Work out the finished part from the listing and answer in its coordinate system (mm). Face numbers are marked on the shaded views. A direction names the side the tool comes from. Coordinates: 2 decimals unless noted, no trailing zeros. Loops run counter-clockwise (first coordinate to the right, second up) from the corner with the lowest first, then second, coordinate; pieces in that order, holes last. Notation, with made-up numbers: M 61,-3.75 L 86,-3.75 A22 cw 86,9.25 Z; hole C 27,-29.5 d2. An arc over 180 degrees is marked long. Write each question's results on one line, items separated by ' | '.
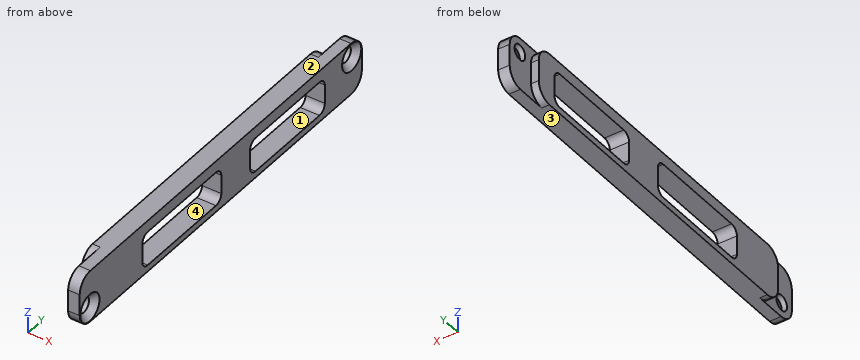
Autodesk Inventor part; units mm, degrees
ref_plane "YZ Plane" through (0, 0, 0) normal (1, 0, 0) x (0, 1, 0)
ref_plane "XZ Plane" through (0, 0, 0) normal (0, 1, 0) x (-1, 0, 0)
ref_plane "XY Plane" through (0, 0, 0) normal (0, 0, 1) x (1, 0, 0)
sketch "Sketch1" plane through (0, 0, 0) normal (1, 0, 0) x (0, 1, 0)
  line L0 (2, 0) -> (50.8, 0)
  line L1 (52.8, -2) -> (52.8, -4.8)
  line L2 (50.8, -6.8) -> (2, -6.8)
  line L3 (0, -4.8) -> (0, -2)
  arc A0 (2, 0) -> (0, -2) centre (2, -2) ccw
  arc A1 (0, -4.8) -> (2, -6.8) centre (2, -4.8) ccw
  arc A2 (50.8, -6.8) -> (52.8, -4.8) centre (50.8, -4.8) ccw
  arc A3 (52.8, -2) -> (50.8, 0) centre (50.8, -2) ccw
  line L4 (26.4, 0) -> (26.4, -6.5481) construction
  line L5 (52.8, -3.4) -> (39.7965, -3.4) construction
  circle A4 centre (1.9, -4.9) radius 1
  circle A5 centre (50.9, -4.9) radius 1 construction
  circle A6 centre (50.9, -1.9) radius 1
  point P0 (0, 0)
  point P1 (52.8, 0)
  point P2 (0, -6.8)
  dimension "d0" = 52.8
  dimension "d1" = 6.8
  dimension "d2" = 2
  dimension "d19" = 2
  dimension "d20" = 0.1
  dimension "d21" = 0.1
extrude "Extrusion1" add sketch "Sketch1" along normal blind 1.5
chamfer "Chamfer1" distance 0.8 angle 45 2 edges at (1.5, 49.9, -1.9) (1.5, 0.9, -4.9)
sketch "Sketch2" plane through (1.5, 0, 0) normal (1, 0, 0) x (0, 0, -1)
  line L0 (0, 50.8) -> (0, 2)
  line L1 (2.5, 45.871) -> (4.9546, 45.871)
  line L2 (5.9546, 44.871) -> (5.9546, 32.8996)
  line L3 (4.9546, 31.8996) -> (2.5, 31.8996)
  line L4 (1.5, 32.8996) -> (1.5, 44.871)
  line L5 (2.5, 26.5) -> (4.9546, 26.5)
  line L6 (5.9546, 25.5) -> (5.9546, 12.7187)
  line L7 (4.9546, 11.7187) -> (2.5, 11.7187)
  line L8 (1.5, 12.7187) -> (1.5, 25.5)
  arc A0 (5.9546, 44.871) -> (4.9546, 45.871) centre (4.9546, 44.871) ccw
  arc A1 (2.5, 45.871) -> (1.5, 44.871) centre (2.5, 44.871) ccw
  arc A2 (1.5, 32.8996) -> (2.5, 31.8996) centre (2.5, 32.8996) ccw
  arc A3 (4.9546, 31.8996) -> (5.9546, 32.8996) centre (4.9546, 32.8996) ccw
  arc A4 (5.9546, 25.5) -> (4.9546, 26.5) centre (4.9546, 25.5) ccw
  arc A5 (4.9546, 11.7187) -> (5.9546, 12.7187) centre (4.9546, 12.7187) ccw
  arc A6 (1.5, 12.7187) -> (2.5, 11.7187) centre (2.5, 12.7187) ccw
  arc A7 (2.5, 26.5) -> (1.5, 25.5) centre (2.5, 25.5) ccw
  point P0 (0, 0)
  dimension "d9" = 1
  dimension "d10" = 1.5
  dimension "d11" = 1.5
extrude "Extrusion2" cut sketch "Sketch2" against normal blind 1.5
sketch "Sketch3" plane through (0, 0, 0) normal (-1, 0, 0) x (0, 0, 1)
  arc A0 (-1.5, 44.871) -> (-2.5, 45.871) centre (-2.5, 44.871) ccw
  line L0 (-1.5, 44.871) -> (-1.5, 32.8996)
  arc A1 (-2.5, 31.8996) -> (-1.5, 32.8996) centre (-2.5, 32.8996) ccw
  line L1 (-2.5, 31.8996) -> (-4.9546, 31.8996)
  arc A2 (-5.9546, 32.8996) -> (-4.9546, 31.8996) centre (-4.9546, 32.8996) ccw
  line L2 (-5.9546, 32.8996) -> (-5.9546, 44.871)
  arc A3 (-4.9546, 45.871) -> (-5.9546, 44.871) centre (-4.9546, 44.871) ccw
  line L3 (-4.9546, 45.871) -> (-2.5, 45.871)
  arc A4 (-4.9546, 26.5) -> (-5.9546, 25.5) centre (-4.9546, 25.5) ccw
  line L4 (-4.9546, 26.5) -> (-2.5, 26.5)
  arc A5 (-1.5, 25.5) -> (-2.5, 26.5) centre (-2.5, 25.5) ccw
  line L5 (-1.5, 25.5) -> (-1.5, 12.7187)
  arc A6 (-2.5, 11.7187) -> (-1.5, 12.7187) centre (-2.5, 12.7187) ccw
  line L6 (-2.5, 11.7187) -> (-4.9546, 11.7187)
  arc A7 (-5.9546, 12.7187) -> (-4.9546, 11.7187) centre (-4.9546, 12.7187) ccw
  line L7 (-5.9546, 12.7187) -> (-5.9546, 25.5)
  line L8 (0, 50.8) -> (0, 2)
  line L9 (-4.8, 52.8) -> (-2, 52.8)
  line L10 (-4.8, 48.8) -> (-2, 48.8)
  line L11 (0, 46.8) -> (0, 6)
  line L12 (-2, 4) -> (-4.8, 4)
  line L13 (-6.8, 6) -> (-6.8, 46.8)
  arc A8 (-4.8, 48.8) -> (-6.8, 46.8) centre (-4.8, 46.8) ccw
  arc A9 (0, 46.8) -> (-2, 48.8) centre (-2, 46.8) ccw
  arc A10 (-2, 4) -> (0, 6) centre (-2, 6) ccw
  arc A11 (-6.8, 6) -> (-4.8, 4) centre (-4.8, 6) ccw
  line L14 (-3.4, 52.8) -> (-3.4, 49.069) construction
  line L15 (-3.4, 48.8) -> (-3.4, 44.871) construction
  line L16 (0, 26.4) -> (-3, 26.4) construction
  line L17 (-6.8, 26.4) -> (-12.1303, 26.4) construction
  point P0 (0, 0)
  point P1 (0, 4)
  point P2 (0, 48.8)
  point P3 (-6.8, 4)
  point P4 (-6.8, 45.8508)
  point P5 (-6.8, 31.9198)
  point P6 (-6.8, 26.4798)
  point P7 (-6.8, 11.7389)
  dimension "d14" = 6.8
  dimension "d15" = 44.8
  dimension "d16" = 2
extrude "Extrusion3" add sketch "Sketch3" along normal blind 1
properties part number "IOModulePlate01"
1) Given pin 1 Ø1.8 at (y, z) = (50, -3.5) entering from -X; pin 2 Ø1.5 at (x, z) = (-0.5, -6) entering from -Y, each flat-ended and moving along its own axis, determine where each tip first touches the part or whether it passes through.
Check result:
pin 1: x = 0 | pin 2: y = 0.11
2) Which of the six approach directions +Z, -Z, +X, -X, +Y, -Y give full straight-line access (tool end or side, diameter ignored) to the marked faces 1 and 2?
Check result:
face 1: +X, -X | face 2: +Z, +X, -X, +Y, -Y
3) For a pull along Y with two mould halves and no side action, classify the marked faces 3 and 4 as released by +Y, released by -Y, zero draft, split by the parting line, or undercut.
Check result:
face 3: zero draft | face 4: undercut
4) Find section A-A, the plane y = 20.5. Give the vertices of the cut face in (x, z).
Check result:
outline: M -1,-6.8 L 1.5,-6.8 L 1.5,-5.95 L -1,-5.95 Z; M -1,-1.5 L 1.5,-1.5 L 1.5,0 L -1,0 Z
5) Straight lines are drawn through the part: probe 1 along Y at (x, z) = (-0.7, -3); probe 2 along Z at (x, y) = (1.1, 43); probe 3 along Z at (x, y) = (0.35, 1.9). For each, find the intervals that lie inside material, in ascending order. Write a range as [from, to].
Check result:
probe 1: [4, 11.72], [26.5, 31.9], [45.87, 48.8] | probe 2: [-6.8, -5.95], [-1.5, 0] | probe 3: [-6.8, -5.9], [-3.9, 0]
6) Find section B-B, the plane x = 1.1. Give the vertices of the cut face in (y, z), and give its area (3 significant figures).
Check result:
outline: M 0,-4.8 A2 ccw 2,-6.8 L 50.8,-6.8 A2 ccw 52.8,-4.8 L 52.8,-2 A2 ccw 50.8,0 L 2,0 A2 ccw 0,-2 Z; hole C 1.9,-4.9 d2.8; hole M 11.72,-4.95 A1 ccw 12.72,-5.95 L 25.5,-5.95 A1 ccw 26.5,-4.95 L 26.5,-2.5 A1 ccw 25.5,-1.5 L 12.72,-1.5 A1 ccw 11.72,-2.5 Z; hole M 31.9,-4.95 A1 ccw 32.9,-5.95 L 44.87,-5.95 A1 ccw 45.87,-4.95 L 45.87,-2.5 A1 ccw 44.87,-1.5 L 32.9,-1.5 A1 ccw 31.9,-2.5 Z; hole C 50.9,-1.9 d2.8 | area: 217 mm^2
